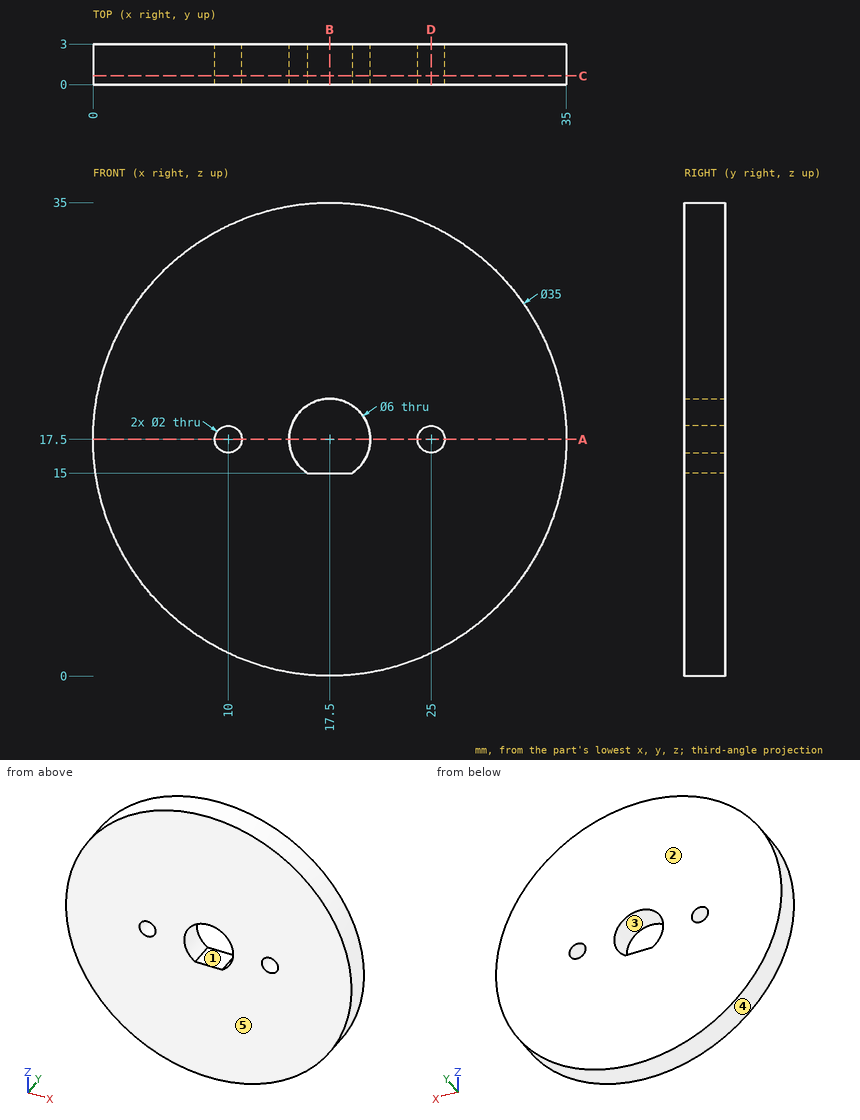
Source: three-view drawing plus pictorial views. Frame: mm from the lowest corner of the part. A direction names the side the tool comes from. Give positions to 0.01 mm unless a question says otherwise; leave off trailing zeros. Order: outer loops, then holes, each group sorted by start corner. A loop starts at its lowest first (then second) coordinate and runs counter-clockwise, first axis right, second up. Notation, with made-up numbers: (-22, -30.75) -> (20, -30.75) arc R13 ccw to (20, -9.75) -> close; hole circle Ø1 at (28.25, 41.25). An arc over 180 degrees is marked (long way). Put each result on its own line as item: value.
Q1. Section C-C, the plane y = 0.65. Return loops of the section in (x, z), then the cut area to 3 significant figures.
Here are the results:
outline: circle Ø35 at (17.5, 17.5); hole circle Ø2 at (10, 17.5); hole (15.84, 15) -> (19.16, 15) arc R3 ccw (long way) to start; hole circle Ø2 at (25, 17.5)
area: 929 mm^2
Q2. Reachability of the marked faces 1 and 2 from +Z, -Z, +X, -X, +Y, -Y: full face, straight path, thin tool, end or side. Return the list, or none.
Here are the results:
face 1: +Y, -Y
face 2: +Z, -Z, +X, -X, +Y
Q3. Section A-A, the plane z = 17.5. Return loops of the section in (x, y).
Here are the results:
outline: (0, 0) -> (9, 0) -> (9, 3) -> (0, 3) -> close; (11, 0) -> (14.5, 0) -> (14.5, 3) -> (11, 3) -> close; (20.5, 0) -> (24, 0) -> (24, 3) -> (20.5, 3) -> close; (26, 0) -> (35, 0) -> (35, 3) -> (26, 3) -> close
Q4. Draft query along X for the marked faces 3, 4 and 5. Return one class per face: released by +X, released by -X, zero draft, split by the parting line, or undercut.
Here are the results:
face 3: undercut
face 4: split by the parting line
face 5: zero draft
Q5. Section D-D, the plane x = 25. Return loops of the section in (y, z).
Here are the results:
outline: (0, 1.69) -> (3, 1.69) -> (3, 16.5) -> (0, 16.5) -> close; (0, 18.5) -> (3, 18.5) -> (3, 33.31) -> (0, 33.31) -> close
Q6. Material intervals for L1, parallel to X at y = 1.1, z = 17.5; L2, parallel to Z at x = 16.5, y = 1; L3, parallel to X at y = 0.3, z = 19, sorted ascending.
Here are the results:
L1: x = 0 to 9, 11 to 14.5, 20.5 to 24, 26 to 35
L2: z = 0.03 to 15, 20.33 to 34.97
L3: x = 0.06 to 14.9, 20.1 to 34.94
Q7. Section B-B, the plane x = 17.5. Return loops of the section in (y, z).
Here are the results:
outline: (0, 0) -> (3, 0) -> (3, 15) -> (0, 15) -> close; (0, 20.5) -> (3, 20.5) -> (3, 35) -> (0, 35) -> close
Q8. Pin query (flat end, axial travel): pin 1 (1.5 mm diameter, centred on y = 2, z = 5.5, fed in from -X); pin 2 (9.5 mm diameter, centred on x = 17.5, z = 17.5, fed in from -Y). Return the tip coordinate at first contact, or that it passes through.
Here are the results:
pin 1: stops at x = 4.1
pin 2: stops at y = 0
